Autodesk Inventor part; units mm, degrees
ref_plane "YZ Plane" through (0, 0, 0) normal (1, 0, 0) x (0, 1, 0)
ref_plane "XZ Plane" through (0, 0, 0) normal (0, 1, 0) x (-1, 0, 0)
ref_plane "XY Plane" through (0, 0, 0) normal (0, 0, 1) x (1, 0, 0)
sketch "Sketch1" plane through (0, 0, 0) normal (0, 1, 0) x (-1, 0, 0)
  point P0 (0, 0)
sketch "Sketch2" plane through (0, 0, 0) normal (0, 1, 0) x (-1, 0, 0)
  line L0 (125, 80) -> (-125, 80)
  line L1 (-125, 80) -> (-125, -80)
  line L2 (-125, -80) -> (125, -80)
  line L3 (125, -80) -> (125, 80)
  point P0 (0, 0)
  dimension "d0" = 250
  dimension "d1" = 160
  dimension "d2" = 80
  dimension "d3" = 125
extrude "Extrusion1" add sketch "Sketch2" along normal blind 4
sketch "Sketch3" plane through (0, 4, 0) normal (0, 1, 0) x (1, 0, 0)
  line L0 (-75, 80) -> (-35, 80)
  line L1 (-35, 80) -> (-35, 50)
  line L2 (-35, 50) -> (-75, 50)
  line L3 (-75, 50) -> (-75, 80)
  line L4 (125, 80) -> (-125, 80)
  line L5 (35, 80) -> (75, 80)
  line L6 (75, 80) -> (75, 50)
  line L7 (75, 50) -> (35, 50)
  line L8 (35, 50) -> (35, 80)
  line L9 (319.9785, -5.3403) -> (359.9785, -5.3403)
  line L10 (359.9785, -5.3403) -> (359.9785, -35.3403)
  line L11 (359.9785, -35.3403) -> (319.9785, -35.3403)
  line L12 (319.9785, -35.3403) -> (319.9785, -5.3403)
  line L13 (-75, -50) -> (-35, -50)
  line L14 (-35, -50) -> (-35, -80)
  line L15 (-35, -80) -> (-75, -80)
  line L16 (-75, -80) -> (-75, -50)
  line L17 (35, -50) -> (75, -50)
  line L18 (75, -50) -> (75, -80)
  line L19 (75, -80) -> (35, -80)
  line L20 (35, -80) -> (35, -50)
  line L21 (-125, -80) -> (125, -80)
  line L22 (-125, 80) -> (-125, -80)
  line L23 (-115, 6) -> (-92, 6)
  line L24 (-92, 6) -> (-92, -6)
  line L25 (-92, -6) -> (-115, -6)
  line L26 (-115, -6) -> (-115, 6)
  point P0 (0, 0)
  point P1 (-35, 65)
  point P2 (-75, 65)
  point P3 (-55, 80)
  point P4 (75, 65)
  point P5 (160.9592, -18.931)
  point P6 (359.9785, -20.3403)
  point P7 (72.8179, -60.7416)
  point P8 (-35, -65)
  point P9 (-133.4102, -90.6871)
  point P10 (75, -65)
  point P11 (55, 80)
  point P12 (35, 65)
  point P13 (35, -65)
  point P14 (55, -80)
  point P15 (-75, -65)
  point P16 (-103.5, -6)
  point P17 (-103.5, 6)
  point P18 (-115, 0)
  point P19 (-92, 0)
  point P20 (-125, 0)
  dimension "d6" = 30
  dimension "d7" = 40
  dimension "d8" = 35
  dimension "d9" = 0
  dimension "d10" = 40
  dimension "d11" = 30
  dimension "d12" = 40
  dimension "d13" = 30
  dimension "d14" = 40
  dimension "d15" = 30
  dimension "d16" = 40
  dimension "d17" = 30
  dimension "d18" = 0
  dimension "d19" = 35
  dimension "d20" = 35
  dimension "d21" = 0
  dimension "d22" = 50
  dimension "d23" = 0
  dimension "d24" = 12
  dimension "d25" = 0
  dimension "d26" = 23
  dimension "d27" = 10
extrude "Extrusion2" cut sketch "Sketch3" against normal blind 10 contours L4 L6 L7 L8 | L0 L1 L2 L3 | L20 L17 L18 L19 | L16 L13 L14 L15 | L23 L24 L25 L26
sketch "Sketch4" plane through (0, 4, 0) normal (0, 1, 0) x (1, 0, 0)
  point P0 (0, 0)
properties part number "Acrylic bottom"
Here's how the part is built. I have some questions about the finished solid (model axes, mm). Give positions to 0.01 mm unless a question says otherwise; leave off trailing zeros. Write each loop counter-clockwise with the first axis right and the second up, starting at its lowest first coordinate (ties: lowest second). Pieces come first, ordered by that corner, then holes. Notation, with made-up numbers: (64, 5) -> (101, 5) arc R18 ccw to (101, 22) -> close; hole circle Ø7 at (58.25, 75). An arc over 180 degrees is marked (long way). Use one line per item in the form item = value. Start each with the question number.
1. Will these pins go through, and if not, where does the flat tip stop? pin 1 Ø2 at (x, y) = (52, 1) entering from -Z; pin 2 Ø2 at (x, y) = (-63.5, 2.5) entering from +Z.
2. Imagine slicing it at A-A on z = -55. List the corners of the cut face in (x, y) for me.
3. If I drill on L1, parallel to X at y = 2.9, z = -54.5; L2, parallel to Z at x = -63, y = 0.75; L3, parallel to Z at x = -103.5, y = 0.45, over which ranges is the centre line in solid material (lowest first)?
4. Imagine slicing it at B-B on y = 1.6. List the corners of the cut face in (x, z) for me, plus the area to 3 significant figures.
Entries:
q1.pin_1 = -50
q1.pin_2 = 50
q2.outline = (-125, 0) -> (-75, 0) -> (-75, 4) -> (-125, 4) -> close; (-35, 0) -> (35, 0) -> (35, 4) -> (-35, 4) -> close; (75, 0) -> (125, 0) -> (125, 4) -> (75, 4) -> close
q3.L1 = -125 to -75, -35 to 35, 75 to 125
q3.L2 = -50 to 50
q3.L3 = -80 to -6, 6 to 80
q4.outline = (-125, -80) -> (-75, -80) -> (-75, -50) -> (-35, -50) -> (-35, -80) -> (35, -80) -> (35, -50) -> (75, -50) -> (75, -80) -> (125, -80) -> (125, 80) -> (75, 80) -> (75, 50) -> (35, 50) -> (35, 80) -> (-35, 80) -> (-35, 50) -> (-75, 50) -> (-75, 80) -> (-125, 80) -> close; hole (-115, -6) -> (-92, -6) -> (-92, 6) -> (-115, 6) -> close
q4.area = 34,900 mm²
